Geometry: see drawing. Coordinates: mm, zero at the bounding-box minimum. A direction names the side the tool comes from. Coordinates: 2 decimals unless noted, no trailing zeros. Order: outer loops, then holes, each group sorted by start corner. A loop starts at its lowest first (then second) coordinate and runs counter-clockwise, first axis right, second up.
Item 1: Mould query, pull axis X, two halves, no side actions, for the marked faces 1, 2, 3 and 4. Classes: released by +X, released by -X, zero draft, split by the parting line, or undercut.
Item 2: Contact query for flat-ended pins moving along their axis: P1, Ø12, axis at x = 24, y = 33.5, coming from the -Z side; P2, Ø2.5, axis at x = 15.5, z = 33, coming from the +Y side; P3, Ø8, axis at x = 4, y = 20.5, coming from the +Z side. Output: stop coordinate, or through.
Item 3: Reachability of the marked faces 5, 6 and 7 from +Z, -Z, +X, -X, +Y, -Y: full face, straight path, thin tool, end or side. Return the list, or none.
Item 4: Section C-C on z = 36. Return the cut outline in (x, y), then the cut area to 3 significant figures.
Item 5: Ray query, line 1 (Y direction, x = 15, z = 27.45); line 2 (Z direction, x = 20.5, y = 35); line 3 (Y direction, x = 2.75, z = 7). Return the intervals inside material, ascending.
Item 6: Section A-A on x = 15. Return the cut outline in (y, z).
Item 7: Section B-B on y = 17.5. Return the cut outline in (x, z).
Item 8: Section D-D on y = 28.5. Return the cut outline in (x, z), then the cut area to 3 significant figures.
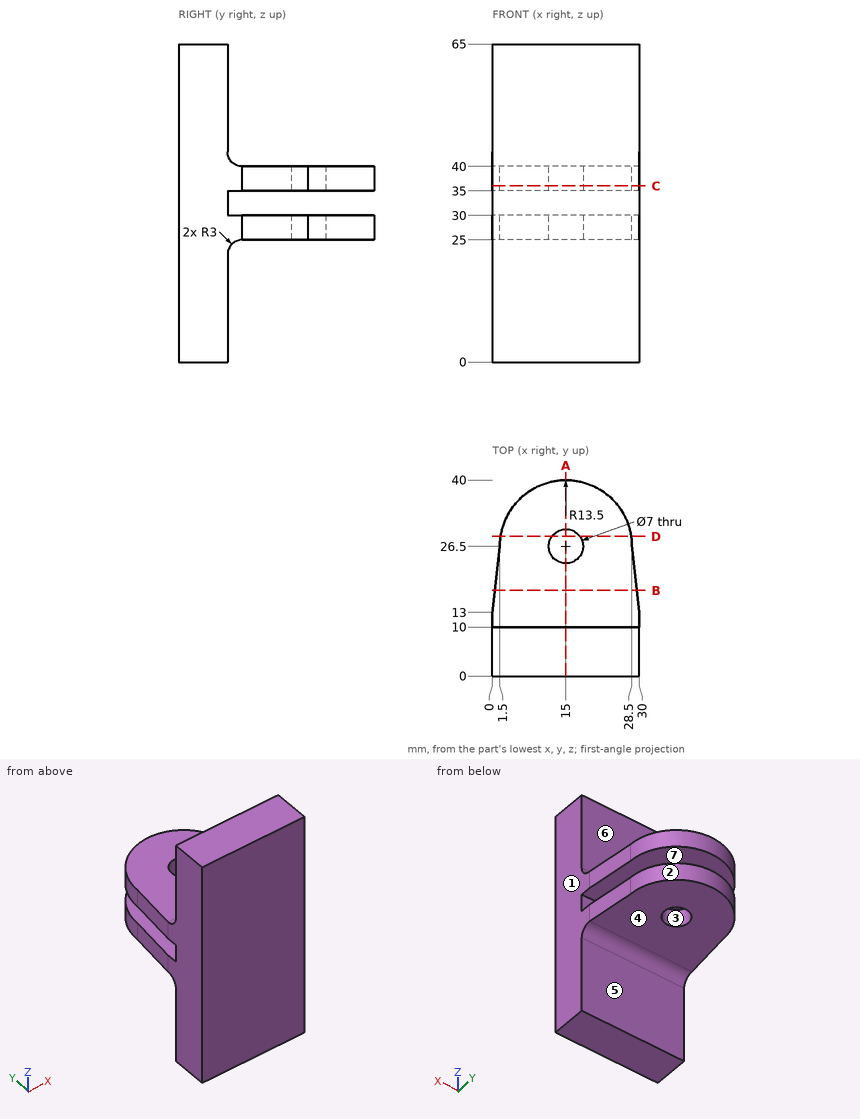
Answer list:
1. face 1: released by +X
1. face 2: split by the parting line
1. face 3: undercut
1. face 4: zero draft
2. P1: stops at z = 25
2. P2: stops at y = 10
2. P3: stops at z = 40
3. face 5: -Z, +X, -X, +Y
3. face 6: +Z, +X, -X, +Y
3. face 7: +X, -X, +Y
4. outline: (0, 0) - (30, 0) - (30, 13) - (28.5, 26.5) arc R13.5 ccw to (1.5, 26.5) - (0, 13) - close; hole circle Ø7 at (15, 26.5)
4. area: 1,020 mm2
5. line 1: y = 0 to 23, 30 to 40
5. line 2: z = 25 to 30, 35 to 40
5. line 3: y = 0 to 10
6. outline: (0, 0) - (10, 0) - (10, 22) arc R3 cw to (13, 25) - (23, 25) - (23, 30) - (10, 30) - (10, 35) - (23, 35) - (23, 40) - (13, 40) arc R3 cw to (10, 43) - (10, 65) - (0, 65) - close; (30, 25) - (40, 25) - (40, 30) - (30, 30) - close; (30, 35) - (40, 35) - (40, 40) - (30, 40) - close
7. outline: (0.5, 25) - (29.5, 25) - (29.5, 30) - (0.5, 30) - close; (0.5, 35) - (29.5, 35) - (29.5, 40) - (0.5, 40) - close
8. outline: (1.65, 25) - (12.13, 25) - (12.13, 30) - (1.65, 30) - close; (1.65, 35) - (12.13, 35) - (12.13, 40) - (1.65, 40) - close; (17.87, 25) - (28.35, 25) - (28.35, 30) - (17.87, 30) - close; (17.87, 35) - (28.35, 35) - (28.35, 40) - (17.87, 40) - close
8. area: 210 mm2
